```python
from build123d import *

# Parameters (mm, degrees)
SKETCH1_W              = 86.9
SKETCH1_H              = 58
BOSS_EXTRUDE1_DEPTH    = 2.5
SKETCH2_R              = 3
BOSS_EXTRUDE2_DEPTH    = 5
LPATTERN1_COUNT        = 2
LPATTERN1_PITCH        = 49
M2_5_CLEARANCE_HOLE1_D = 2.7
SKETCH6_W              = 6.75
SKETCH6_H              = 58
BOSS_EXTRUDE3_DEPTH    = 9.5
SKETCH7_W              = 2.5
SKETCH7_H              = 58
BOSS_EXTRUDE4_DEPTH    = 8
SKETCH8_W              = 2.5
SKETCH8_H              = 58
BOSS_EXTRUDE5_DEPTH    = 8
SKETCH9_R              = 3.15
CUT_EXTRUDE1_DEPTH     = 2.7


with BuildPart() as part:
    # Sketch1 → Boss-Extrude1 (new body)
    with BuildSketch(Plane.XY):
        Rectangle(SKETCH1_W, SKETCH1_H)
    extrude(amount=BOSS_EXTRUDE1_DEPTH)

    # Sketch2 → Boss-Extrude2 (add)
    with BuildSketch(Plane.XY.offset(2.5)):
        with Locations(Location((-29.45, 25.5, 0), (0, 0, 180))):
            Circle(SKETCH2_R)
        with Locations(Location((28.55, 25.5, 0), (0, 0, 180))):
            Circle(SKETCH2_R)
    boss_extrude2 = extrude(amount=BOSS_EXTRUDE2_DEPTH)

    # LPattern1: Boss-Extrude2 ×2
    with Locations(*[(0, -i * LPATTERN1_PITCH, 0) for i in range(1, LPATTERN1_COUNT)]):
        add(boss_extrude2)

    # M2.5 Clearance Hole1 (through all)
    with Locations(Plane.XY.offset(7.5)):
        with Locations((-29.45, 25.5), (-29.45, -23.5), (28.55, 25.5), (28.55, -23.5)):
            Hole(M2_5_CLEARANCE_HOLE1_D / 2)

    # Sketch6 → Boss-Extrude3 (add)
    with BuildSketch(Plane(origin=(0, 0, 0), x_dir=(-1, 0, 0), z_dir=(0, 0, -1))):
        with Locations((-40.075, 0)):
            Rectangle(SKETCH6_W, SKETCH6_H)
        with Locations((40.075, 0)):
            Rectangle(SKETCH6_W, SKETCH6_H)
    extrude(amount=BOSS_EXTRUDE3_DEPTH)

    # Sketch7 → Boss-Extrude4 (add)
    with BuildSketch(Plane.ZY.offset(-36.7)):
        with Locations((-8.25, 0)):
            Rectangle(SKETCH7_W, SKETCH7_H)
    extrude(amount=BOSS_EXTRUDE4_DEPTH)

    # Sketch8 → Boss-Extrude5 (add)
    with BuildSketch(Plane(origin=(-36.7, 0, 0), x_dir=(0, 0, -1), z_dir=(1, 0, 0))):
        with Locations((8.25, 0)):
            Rectangle(SKETCH8_W, SKETCH8_H)
    extrude(amount=BOSS_EXTRUDE5_DEPTH)

    # Sketch9 → Cut-Extrude1 (cut)
    with BuildSketch(Plane.XZ.offset(29)):
        with Locations(Location((-40.075, -3.5, 0), (0, 0, 270))):
            Circle(SKETCH9_R)
        with Locations(Location((40.075, -3.5, 0), (0, 0, 270))):
            Circle(SKETCH9_R)
    extrude(amount=-CUT_EXTRUDE1_DEPTH, mode=Mode.SUBTRACT)


solid = part.part
```
For this review, take the finished solid that the model builds, in its own axes (mm). A direction names the side the tool comes from. Give positions to 0.01 mm unless a question says otherwise; leave off trailing zeros. Write each loop counter-clockwise with the first axis right and the second up, starting at its lowest first coordinate (ties: lowest second). Pieces come first, ordered by that corner, then holes.
Item 1: Take a section at B-B (z = -2.75). Give the boundary of the cut face in (x, y).
Item 2: Machinability: for faces 5 (the face through (33, 0, -7)), 6 (the face through (-30, -22, 7.5)), 7 (the face through (-28.7, 0, -8)), 8 (the face through (-1, 0, 2.5)), 9 (the face through (-40, -26.3, -3)), which of the approach directions +Z, -Z, +X, -X, +Y, -Y give a long, thin tool a straight path to every point of the face, cutting with its end or side? Answer none if there is none.
Item 3: Take a section at A-A (y = 25.5). Give the boundary of the cut face in (x, z), and give its area (3 significant figures).
Item 4: Take a section at C-C (y = -6.5). Give the boundary of the cut face in (x, z).
Item 5: Take a section at D-D (x = -1). Give the boundary of the cut face in (y, z), and give its area (3 significant figures).
Item 6: Insertion check: P1, Ø7, axis at x = 40.075, z = -3.5, coming from the -Y side; P2, Ø6.5, axis at x = -34, y = 11.5, coming from the +Z side; P3, Ø2, axis at x = 28.55, y = -23.5, coming from the +Z side; P4, Ø8, axis at x = 23.5, y = -20.5, coming from the -Z side. Each pin has a flat end and moves straight along its axis. Give the tip position at first contact, or say it passes through.
Item 7: The part is to be moulded in two halves that separate along X. For faces 1 (the face through (31.547, -23.632, 4.965)), 2 (the face through (28, 27, 7.5)), 3 (the face through (-43.45, 0, -4)), 4 (the face through (-33, 0, -7)), say which applies: +X half, -X half, draft (parallel to the pull), parting line (faces both ways), or undercut.
Item 8: Wall thickness on probe 1 along X at (y, z) = (-27.7, -3.5) (3 decimals); probe 2 along Y at (x, z) = (-29.45, 2); probe 3 along X at (y, z) = (-5.5, -0.5): over which ranges is each line inside the solid? List them lowest first.
Established:
1. outline: (-43.45, -29) - (-43.13, -29) - (-43.13, -26.3) - (-37.02, -26.3) - (-37.02, -29) - (-36.7, -29) - (-36.7, 29) - (-43.45, 29) - close; (36.7, -29) - (37.02, -29) - (37.02, -26.3) - (43.13, -26.3) - (43.13, -29) - (43.45, -29) - (43.45, 29) - (36.7, 29) - close
2. face 5: +Y, -Y
2. face 6: +Z, +X, -X, +Y, -Y
2. face 7: -Z, +Y, -Y
2. face 8: +Z
2. face 9: -Y
3. outline: (-43.45, -9.5) - (-28.7, -9.5) - (-28.7, -7) - (-36.7, -7) - (-36.7, 0) - (-30.8, 0) - (-30.8, 7.5) - (-32.45, 7.5) - (-32.45, 2.5) - (-43.45, 2.5) - close; (-28.1, 0) - (27.2, 0) - (27.2, 7.5) - (25.55, 7.5) - (25.55, 2.5) - (-26.45, 2.5) - (-26.45, 7.5) - (-28.1, 7.5) - close; (28.7, -9.5) - (43.45, -9.5) - (43.45, 2.5) - (31.55, 2.5) - (31.55, 7.5) - (29.9, 7.5) - (29.9, 0) - (36.7, 0) - (36.7, -7) - (28.7, -7) - close
3. area: 405 mm2
4. outline: (-43.45, -9.5) - (-28.7, -9.5) - (-28.7, -7) - (-36.7, -7) - (-36.7, 0) - (36.7, 0) - (36.7, -7) - (28.7, -7) - (28.7, -9.5) - (43.45, -9.5) - (43.45, 2.5) - (-43.45, 2.5) - close
5. outline: (-29, 0) - (29, 0) - (29, 2.5) - (-29, 2.5) - close
5. area: 145 mm2
6. P1: stops at y = -29
6. P2: stops at z = 2.5
6. P3: stops at z = -7
6. P4: stops at z = 0
7. face 1: undercut
7. face 2: draft
7. face 3: -X half
7. face 4: undercut
8. probe 1: x = -43.45 to -43.225, -36.925 to -36.7, 36.7 to 36.925, 43.225 to 43.45
8. probe 2: y = -29 to -24.85, -22.15 to 24.15, 26.85 to 29
8. probe 3: x = -43.45 to -36.7, 36.7 to 43.45
